Input: part model. Units: mm. Frame: model coordinates. A direction names the side the tool comes from. Round coordinates to 2 decimals unless told otherwise and drop trailing zeros. Loops run counter-clockwise (first coordinate to the right, second up) from the corner with the lowest first, then second, coordinate; pieces in that order, holes last. Notation, with made-up numbers: (61.5, 11.25) -> (92.5, 11.25) arc R36 cw to (92.5, 46.25) -> close; hole circle Ø7 at (48, 79). An arc over 180 degrees is marked (long way). Answer as a JSON object with one key per item and string values.
```python
from build123d import *

# Parameters (mm, degrees)
CHAMFER_1_SIZE           = 0.5
HOLE_WIZARD_M31_D        = 3.6
PATTERN_CIRCULAR_1_COUNT = 4


with BuildPart() as part:
    # Эскиз1 → Повернуть1 (revolve)
    with BuildSketch(Plane.XY, mode=Mode.PRIVATE) as revolve_1_sk:
        Polygon((-15, 2), (-15, 16), (-26, 16), (-26, 9), (-18, 9), (-18, 0), (-13, 0), (-13, 2), align=None)
    revolve(revolve_1_sk.sketch.rotate(Axis((0, 0, 0), (0, 1, 0)), 270), axis=Axis((0, 0, 0), (0, 1, 0)))

    # Фаска1
    chamfer_1_edges = [part.edges().sort_by_distance(p)[0] for p in [
        (0, 0, 18),
    ]]
    chamfer(chamfer_1_edges, length=CHAMFER_1_SIZE)

    # Отверстие с зазором M31 (through all)
    with Locations(Plane(origin=(0, 16, 0), x_dir=(1, 0, 0), z_dir=(0, 1, 0))):
        with Locations((15.556349186, -15.556349186)):
            hole_wizard_m31 = Hole(HOLE_WIZARD_M31_D / 2)

    # Круговой массив1: Отверстие с зазором M31 ×4 about axis
    pattern_circular_1_axis = Axis((0, 0, 0), (0, 1, 0))
    for i in range(1, PATTERN_CIRCULAR_1_COUNT):
        add(hole_wizard_m31.rotate(pattern_circular_1_axis, i * 360 / PATTERN_CIRCULAR_1_COUNT), mode=Mode.SUBTRACT)


solid = part.part
```
1) Reachability of faces 1 (the face through (-13.4, 2, -0.1)), 2 (the face through (-18, 9, -5)), 3 (the face through (-13.84, 12.45, -15.02)) from +Z, -Z, +X, -X, +Y, -Y: full face, straight path, thin tool, end or side. Return the list, or none.
Output:
{"face 1": "+Y", "face 2": "-Y", "face 3": "+Y, -Y"}
2) Section A-A, the plane x = 0. Output: boundary loops of the cut face in (y, z), plus the area to 3 significant figures.
Output:
{"outline": "(0, -17.5) -> (0.5, -18) -> (9, -18) -> (9, -26) -> (16, -26) -> (16, -15) -> (2, -15) -> (2, -13) -> (0, -13) -> close; (0, 13) -> (2, 13) -> (2, 15) -> (16, 15) -> (16, 26) -> (9, 26) -> (9, 18) -> (0.5, 18) -> (0, 17.5) -> close", "area": "216 mm^2"}
3) Section B-B, the plane z = 0. Output: boundary loops of the cut face in (x, y).
Output:
{"outline": "(-26, 9) -> (-18, 9) -> (-18, 0.5) -> (-17.5, 0) -> (-13, 0) -> (-13, 2) -> (-15, 2) -> (-15, 16) -> (-26, 16) -> close; (13, 0) -> (17.5, 0) -> (18, 0.5) -> (18, 9) -> (26, 9) -> (26, 16) -> (15, 16) -> (15, 2) -> (13, 2) -> close"}
4) Section C-C, the plane y = 4. Output: boundary loops of the cut face in (x, z), plus the area to 3 significant figures.
Output:
{"outline": "circle Ø36 at (0, 0); hole circle Ø30 at (0, 0)", "area": "311 mm^2"}
5) Section D-D, the plane y = 10. Output: boundary loops of the cut face in (x, z).
Output:
{"outline": "circle Ø52 at (0, 0); hole circle Ø3.6 at (-15.56, -15.56); hole circle Ø3.6 at (-15.56, 15.56); hole circle Ø30 at (0, 0); hole circle Ø3.6 at (15.56, -15.56); hole circle Ø3.6 at (15.56, 15.56)"}
6) Draft query along X for faces 4 (the face through (15.821, 12.451, 20.633)), 5 (the face through (7.91, 1.014, 10.316)), 6 (the face through (-13, 0, 3)). Return one class per face: +X half, -X half, draft (parallel to the pull), parting line (faces both ways), or undercut.
Output:
{"face 4": "parting line", "face 5": "undercut", "face 6": "draft"}
7) Ray query, probe 1 along Y at (x, z) = (-17.5, 11); probe 2 along X at (y, z) = (11.5, 11); probe 3 along Z at (x, y) = (-8, 10.75). Return the intervals inside material, ascending.
Output:
{"probe 1": "y = 9 to 16", "probe 2": "x = -23.56 to -10.2, 10.2 to 23.56", "probe 3": "z = -24.74 to -12.69, 12.69 to 24.74"}
8) Contact query for flat-ended pins moving along their axis: P1, Ø8, axis at x = 7.5, z = -11, coming from the -Y side; P2, Ø3, axis at x = -11.5, z = 5.5, coming from the +Y side; P3, Ø3, axis at x = -6, y = 10.5, coming from the -Z side; P4, Ø8, axis at x = 17.5, y = 2, coming from the -Z side. Output: stop coordinate, or through.
Output:
{"P1": "stops at y = 0", "P2": "stops at y = 2", "P3": "stops at z = -25.61", "P4": "stops at z = -11.91"}
